from build123d import *

# Parameters (mm, degrees)
SKETCH_1_W                = 58.8
SKETCH_1_H                = 32
EXTRUDE_1_DEPTH           = 41.5
HOLE_WIZARD_1_D           = 3.2
HOLE_WIZARD_1_CBORE_D     = 6
HOLE_WIZARD_1_CBORE_DEPTH = 32.5
SKETCH_8_R                = 2.6
CUT_EXTRUDE_6_DEPTH       = 33.5
SKETCH_10_W               = 58.8
SKETCH_10_H               = 41.5
EXTRUDE_2_DEPTH           = 3
SKETCH_18_R               = 2.6
CUT_EXTRUDE_14_DEPTH      = 4
SKETCH_19_W               = 20
SKETCH_19_H               = 20
SKETCH_19_R               = 3
CUT_EXTRUDE_15_DEPTH      = 22
SKETCH_20_R               = 3
CUT_EXTRUDE_16_DEPTH      = 5
CUT_EXTRUDE_17_DEPTH      = 6
SKETCH_22_W               = 27.4
SKETCH_22_H               = 21.5
CUT_EXTRUDE_18_DEPTH      = 36
SKETCH_23_R               = 2.6
CUT_EXTRUDE_19_DEPTH      = 16
CUT_EXTRUDE_20_DEPTH      = 6
SKETCH_25_W               = 20
SKETCH_25_H               = 17
SKETCH_25_R               = 2.6
CUT_EXTRUDE_21_DEPTH      = 0.1
SKETCH_27_W               = 17
SKETCH_27_H               = 20.1
CUT_EXTRUDE_22_DEPTH      = 0.1
SKETCH_28_R               = 2.6
CUT_EXTRUDE_23_DEPTH      = 39.7
SKETCH_29_R               = 4.5
SKETCH_29_R_2             = 2.6
CUT_EXTRUDE_24_DEPTH      = 5
SKETCH_30_R               = 2.6
CUT_EXTRUDE_25_DEPTH      = 36.0000001
SKETCH_31_R               = 2.6
EXTRUDE_3_DEPTH           = 35
SKETCH_32_W               = 20.1
SKETCH_32_H               = 17
SKETCH_32_R               = 2.6
CUT_EXTRUDE_26_DEPTH      = 7
SKETCH_33_W               = 20.1
SKETCH_33_H               = 7
SKETCH_33_R               = 3
EXTRUDE_4_DEPTH           = 17
SKETCH_34_R               = 4.5
EXTRUDE_5_DEPTH           = 5
SKETCH_35_R               = 2.6
EXTRUDE_6_DEPTH           = 6.3
SKETCH_39_R               = 2.6
CUT_EXTRUDE_29_DEPTH      = 8
SKETCH_40_W               = 20.1
SKETCH_40_H               = 17
SKETCH_40_R               = 2.6
EXTRUDE_7_DEPTH           = 7.9
SKETCH_41_W               = 20.1
SKETCH_41_H               = 17
CUT_EXTRUDE_30_DEPTH      = 7.9
SKETCH_42_R               = 2.6
CUT_EXTRUDE_31_DEPTH      = 39.7
SKETCH_43_R               = 4.5
SKETCH_43_R_2             = 2.6
CUT_EXTRUDE_32_DEPTH      = 5.2
SKETCH_44_R               = 2.6
EXTRUDE_8_DEPTH           = 3
SKETCH_46_R               = 4.75
SKETCH_46_R_2             = 2.6
CUT_EXTRUDE_33_DEPTH      = 3


with BuildPart() as part:
    # 草图1 → 凸台-拉伸1 (new body)
    with BuildSketch(Plane.XY):
        with Locations((-0.739622642, 3.045283019)):
            Rectangle(SKETCH_1_W, SKETCH_1_H)
    extrude(amount=EXTRUDE_1_DEPTH)

    # 孔1 (through all)
    with Locations(Plane(origin=(11.760377358, 15.545283019, 0), x_dir=(-1, 0, 0), z_dir=(0, 0, -1))):
        with Locations((0, 0), (25, 0), (25, -25), (0, -25)):
            CounterBoreHole(HOLE_WIZARD_1_D / 2, HOLE_WIZARD_1_CBORE_D / 2, HOLE_WIZARD_1_CBORE_DEPTH)

    # 草图8 → 切除-拉伸6 (cut)
    with BuildSketch(Plane(origin=(0, 19.045283019, 0), x_dir=(1, 0, 0), z_dir=(0, 1, 0))):
        with Locations((-0.739622642, -31.5)):
            Circle(SKETCH_8_R)
    extrude(amount=-CUT_EXTRUDE_6_DEPTH, mode=Mode.SUBTRACT)

    # 草图10 → 凸台-拉伸2 (add)
    with BuildSketch(Plane.XZ.offset(12.954716981)):
        with Locations((-0.739622642, 20.75)):
            Rectangle(SKETCH_10_W, SKETCH_10_H)
    extrude(amount=EXTRUDE_2_DEPTH)

    # 草图18 → 切除-拉伸14 (cut, through all)
    with BuildSketch(Plane(origin=(0, -12.954716981, 0), x_dir=(1, 0, 0), z_dir=(0, 1, 0))):
        with Locations((-0.739622642, -31.5)):
            Circle(SKETCH_18_R)
    extrude(amount=-CUT_EXTRUDE_14_DEPTH, mode=Mode.SUBTRACT)

    # 草图19 → 切除-拉伸15 (cut)
    with BuildSketch(Plane(origin=(0, 0, 0), x_dir=(-1, 0, 0), z_dir=(0, 0, -1))):
        with Locations((20.139622642, 9.045283019)):
            Rectangle(SKETCH_19_W, SKETCH_19_H)
        with Locations((13.239622642, 15.545283019)):
            Circle(SKETCH_19_R, mode=Mode.SUBTRACT)
    extrude(amount=-CUT_EXTRUDE_15_DEPTH, mode=Mode.SUBTRACT)

    # 草图20 → 切除-拉伸16 (cut)
    with BuildSketch(Plane(origin=(0, 0, 0), x_dir=(-1, 0, 0), z_dir=(0, 0, -1))):
        Polygon((30.139622642, -15.954716981), (30.139622642, -0.954716981), (10.139622642, -0.954716981), (10.139622642, 19.045283019), (-28.660377358, 19.045283019), (-28.660377358, -15.954716981), align=None)
        with Locations((13.239622642, -9.454716981)):
            Circle(SKETCH_20_R, mode=Mode.SUBTRACT)
        with Locations((-11.760377358, -9.454716981)):
            Circle(SKETCH_20_R, mode=Mode.SUBTRACT)
        with Locations((-11.760377358, 15.545283019)):
            Circle(SKETCH_20_R, mode=Mode.SUBTRACT)
    extrude(amount=-CUT_EXTRUDE_16_DEPTH, mode=Mode.SUBTRACT)

    # 草图21 → 切除-拉伸17 (cut)
    with BuildSketch(Plane.XZ.offset(15.954716981)):
        Polygon((-30.139622642, 19.214629022), (-17.064744213, 5), (-30.139622642, 5), align=None)
    extrude(amount=-CUT_EXTRUDE_17_DEPTH, mode=Mode.SUBTRACT)

    # 草图22 → 切除-拉伸18 (cut, through all)
    with BuildSketch(Plane(origin=(0, 19.045283019, 0), x_dir=(1, 0, 0), z_dir=(0, 1, 0))):
        with Locations((14.960377358, -15.75)):
            Rectangle(SKETCH_22_W, SKETCH_22_H)
    extrude(amount=-CUT_EXTRUDE_18_DEPTH, mode=Mode.SUBTRACT)

    # 草图23 → 切除-拉伸19 (cut, through all)
    with BuildSketch(Plane(origin=(0, -0.954716981, 0), x_dir=(1, 0, 0), z_dir=(0, 1, 0))):
        with Locations((-20.139622642, -13.5)):
            Circle(SKETCH_23_R)
    extrude(amount=-CUT_EXTRUDE_19_DEPTH, mode=Mode.SUBTRACT)

    # 草图24 → 切除-拉伸20 (cut)
    with BuildSketch(Plane(origin=(0, -15.954716981, 0), x_dir=(-1, 0, 0), z_dir=(0, -1, 0))):
        with BuildLine():
            ThreePointArc((20.787086214, -9.046822379), (16.827633547, -16.546428767), (24.631280369, -13.22611889))
            Line((24.631280369, -13.22611889), (20.787086214, -9.046822379))
        make_face()
        with BuildLine():
            ThreePointArc((20.139622642, -16.1), (18.30114501, -11.661522369), (22.739622642, -13.5))
            ThreePointArc((22.739622642, -13.5), (21.978100273, -15.338477631), (20.139622642, -16.1))
        make_face(mode=Mode.SUBTRACT)
    extrude(amount=-CUT_EXTRUDE_20_DEPTH, mode=Mode.SUBTRACT)

    # 草图25 → 切除-拉伸21 (cut)
    with BuildSketch(Plane(origin=(0, -0.954716981, 0), x_dir=(1, 0, 0), z_dir=(0, 1, 0))):
        with Locations((-20.139622642, -13.5)):
            Rectangle(SKETCH_25_W, SKETCH_25_H)
        with Locations((-20.139622642, -13.5)):
            Circle(SKETCH_25_R, mode=Mode.SUBTRACT)
    extrude(amount=-CUT_EXTRUDE_21_DEPTH, mode=Mode.SUBTRACT)

    # 草图27 → 切除-拉伸22 (cut)
    with BuildSketch(Plane.ZY.offset(10.139622642)):
        with Locations((13.5, 8.995283019)):
            Rectangle(SKETCH_27_W, SKETCH_27_H)
    extrude(amount=-CUT_EXTRUDE_22_DEPTH, mode=Mode.SUBTRACT)

    # 草图28 → 切除-拉伸23 (cut, through all)
    with BuildSketch(Plane.ZY.offset(10.039622642)):
        with Locations((13.5, 8.995283019)):
            Circle(SKETCH_28_R)
    extrude(amount=-CUT_EXTRUDE_23_DEPTH, mode=Mode.SUBTRACT)

    # 草图29 → 切除-拉伸24 (cut)
    with BuildSketch(Plane(origin=(1.260377358, 0, 0), x_dir=(0, 0, -1), z_dir=(1, 0, 0))):
        with Locations((-13.5, 8.995283019)):
            Circle(SKETCH_29_R)
        with Locations((-13.5, 8.995283019)):
            Circle(SKETCH_29_R_2, mode=Mode.SUBTRACT)
    extrude(amount=-CUT_EXTRUDE_24_DEPTH, mode=Mode.SUBTRACT)

    # 草图30 → 切除-拉伸25 (cut, through all)
    with BuildSketch(Plane(origin=(0, 19.045283019, 0), x_dir=(1, 0, 0), z_dir=(0, 1, 0))):
        with Locations((-20.139622642, -31.5)):
            Circle(SKETCH_30_R)
    extrude(amount=-CUT_EXTRUDE_25_DEPTH, mode=Mode.SUBTRACT)

    # 草图31 → 凸台-拉伸3 (add, through all)
    with BuildSketch(Plane(origin=(0, 19.045283019, 0), x_dir=(1, 0, 0), z_dir=(0, 1, 0))):
        with Locations((-0.739622642, -31.5)):
            Circle(SKETCH_31_R)
    extrude(amount=-EXTRUDE_3_DEPTH)

    # 草图32 → 切除-拉伸26 (cut)
    with BuildSketch(Plane(origin=(0, -1.054716981, 0), x_dir=(1, 0, 0), z_dir=(0, 1, 0))):
        with Locations((-20.089622642, -13.5)):
            Rectangle(SKETCH_32_W, SKETCH_32_H)
        with Locations((-20.139622642, -13.5)):
            Circle(SKETCH_32_R, mode=Mode.SUBTRACT)
    extrude(amount=-CUT_EXTRUDE_26_DEPTH, mode=Mode.SUBTRACT)

    # 草图33 → 凸台-拉伸4 (add)
    with BuildSketch(Plane(origin=(0, 0, 22), x_dir=(-1, 0, 0), z_dir=(0, 0, -1))):
        with Locations((20.089622642, 15.545283019)):
            Rectangle(SKETCH_33_W, SKETCH_33_H)
        with Locations((13.239622642, 15.545283019)):
            Circle(SKETCH_33_R, mode=Mode.SUBTRACT)
    extrude(amount=EXTRUDE_4_DEPTH)

    # 草图34 → 凸台-拉伸5 (add)
    with BuildSketch(Plane(origin=(-3.739622642, 0, 0), x_dir=(0, 0, -1), z_dir=(1, 0, 0))):
        with Locations((-13.5, 8.995283019)):
            Circle(SKETCH_34_R)
    extrude(amount=EXTRUDE_5_DEPTH)

    # 草图35 → 凸台-拉伸6 (add)
    with BuildSketch(Plane.ZY.offset(3.739622642)):
        with Locations((13.5, 8.995283019)):
            Circle(SKETCH_35_R)
    extrude(amount=EXTRUDE_6_DEPTH)

    # 草图39 → 切除-拉伸29 (cut, through all)
    with BuildSketch(Plane.XZ.offset(-12.045283019)):
        with Locations((-20.139622642, 13.5)):
            Circle(SKETCH_39_R)
    extrude(amount=-CUT_EXTRUDE_29_DEPTH, mode=Mode.SUBTRACT)

    # 草图40 → 凸台-拉伸7 (add)
    with BuildSketch(Plane.XZ.offset(-12.045283019)):
        with Locations((-20.089622642, 13.5)):
            Rectangle(SKETCH_40_W, SKETCH_40_H)
        with Locations((-20.139622642, 13.5)):
            Circle(SKETCH_40_R, mode=Mode.SUBTRACT)
    extrude(amount=EXTRUDE_7_DEPTH)

    # 草图41 → 切除-拉伸30 (cut)
    with BuildSketch(Plane(origin=(0, -8.054716981, 0), x_dir=(1, 0, 0), z_dir=(0, 1, 0))):
        with Locations((-20.089622642, -13.5)):
            Rectangle(SKETCH_41_W, SKETCH_41_H)
    extrude(amount=-CUT_EXTRUDE_30_DEPTH, mode=Mode.SUBTRACT)

    # 草图42 → 切除-拉伸31 (cut, through all)
    with BuildSketch(Plane.ZY.offset(10.039622642)):
        with Locations((13.5, -5.854716981)):
            Circle(SKETCH_42_R)
    extrude(amount=-CUT_EXTRUDE_31_DEPTH, mode=Mode.SUBTRACT)

    # 草图43 → 切除-拉伸32 (cut)
    with BuildSketch(Plane(origin=(1.260377358, 0, 0), x_dir=(0, 0, -1), z_dir=(1, 0, 0))):
        with Locations((-13.5, -5.854716981)):
            Circle(SKETCH_43_R)
        with Locations((-13.5, -5.854716981)):
            Circle(SKETCH_43_R_2, mode=Mode.SUBTRACT)
    extrude(amount=-CUT_EXTRUDE_32_DEPTH, mode=Mode.SUBTRACT)

    # 草图44 → 凸台-拉伸8 (add)
    with BuildSketch(Plane(origin=(0, 19.045283019, 0), x_dir=(1, 0, 0), z_dir=(0, 1, 0))):
        Polygon((1.260377358, -5), (-30.139622642, -5), (-30.139622642, -41.5), (28.660377358, -41.5), (28.660377358, -26.5), (1.260377358, -26.5), align=None)
        with Locations((-20.139622642, -13.5)):
            Circle(SKETCH_44_R, mode=Mode.SUBTRACT)
        with Locations((-20.139622642, -31.5)):
            Circle(SKETCH_44_R, mode=Mode.SUBTRACT)
    extrude(amount=EXTRUDE_8_DEPTH)

    # 草图46 → 切除-拉伸33 (cut)
    with BuildSketch(Plane(origin=(0, 22.045283019, 0), x_dir=(1, 0, 0), z_dir=(0, 1, 0))):
        with Locations((-20.139622642, -31.5)):
            Circle(SKETCH_46_R)
        with Locations((-20.139622642, -31.5)):
            Circle(SKETCH_46_R_2, mode=Mode.SUBTRACT)
    extrude(amount=-CUT_EXTRUDE_33_DEPTH, mode=Mode.SUBTRACT)


solid = part.part
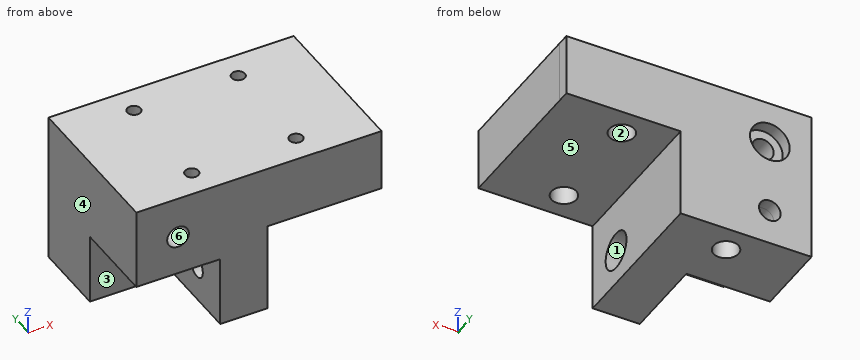
Work out the finished part from the listing and answer in its coordinate system (mm). Face numbers are marked on the shaded views. A direction names the side the tool comes from. Coordinates: 2 decimals unless noted, no trailing zeros. Write each loop counter-clockwise with the first axis right and the second up, starting at its lowest first coordinate (ties: lowest second). Pieces come first, ordered by that corner, then holes. Notation, with made-up numbers: M 63,25.5 L 121,25.5 A35 ccw 121,60.5 Z; hole C 57.5,67 d3. An arc over 180 degrees is marked long. Answer as CSV lines item,"result". Start each with the question number.
Item 1: Consider L1, parallel to X at y = 20, z = 13.5; L2, parallel to Y at x = -11.5, z = 28; L3, parallel to Z at x = -11, y = 16.5. Determine where each line is inside the solid, lowest interval first.
Item 2: Determine the mould class of the marked faces 4, 5 and 6 for opening direction X: released by +X, released by -X, zero draft, split by the parting line, or undercut.
Item 3: A tool of negligible diameter and unlimited length cuts with its end or side. For the marked faces 1, 2 and 3, from which of +Z, -Z, +X, -X, +Y, -Y can it reach the whole face along a straight path? Write none if from no direction.
Item 4: Section C-C on y = 2.5 is taken. Write down the section's boundary in (x, z).
Item 5: Section D-D on z = 31.5 is taken. Write down the section's boundary in (x, y), and give its area (3 significant figures).
Item 6: Flat-ended cylindrical pins translate along their axes: P1, Ø1.5, axis at x = 8.5, y = 1.5, coming from the -Z side; P2, Ø1.9, axis at x = -13.24, y = 15.55, coming from the -Z side; P3, Ø18.5, axis at y = -6, z = 10.5, coming from the -X side; P4, Ø1.8, axis at x = 12.5, y = 14.5, coming from the -Z side. Find the tip coordinate at first contact, or state that the pin passes through.
Item 7: Section B-B on z = 13.5 is taken. Write down the section's boundary in (x, y), and give its area (3 significant figures).
Item 8: Section A-A on y = -4 is taken. Write down the section's boundary in (x, z), and give its area (3 significant figures).
Checks:
1,L1,"x = -30.14 to -22.74, -17.54 to 1.26"
1,L2,"y = -15.95 to -11.9, -7.01 to 13.1, 17.99 to 22.05"
1,L3,"z = 32.5 to 41.5"
2,face 4,"released by -X"
2,face 5,"zero draft"
2,face 6,"undercut"
3,face 1,"+X"
3,face 2,"-Z"
3,face 3,"-Z, -X, -Y"
4,outline,"M -30.14,22 L -10.04,22 L -10.04,5 L 1.26,5 L 1.26,26.5 L 28.66,26.5 L 28.66,41.5 L -30.14,41.5 Z; hole C -20.14,31.5 d5.2"
5,outline,"M -30.14,-15.95 L -22.74,-15.95 L -22.74,19.05 L -24.89,19.05 L -24.89,22.05 L -30.14,22.05 Z; M -17.54,-15.95 L 28.66,-15.95 L 28.66,22.05 L -15.39,22.05 L -15.39,19.05 L -17.54,19.05 Z; hole C -13.24,-9.45 d6; hole C -13.24,15.55 d6; hole C 11.76,-9.45 d6; hole C 11.76,15.55 d6"
5,area,"1,910 mm²"
6,P1,"stops at z = 26.5"
6,P2,"passes through"
6,P3,"stops at x = -10.04"
6,P4,"stops at z = 32.5"
7,outline,"M -30.14,4.15 L -22.74,4.15 L -22.74,22.05 L -30.14,22.05 Z; M -17.54,4.15 L -10.04,4.15 L -10.04,-3.25 L -3.94,-3.25 L -3.94,-1.35 L 1.26,-1.35 L 1.26,22.05 L -17.54,22.05 Z; M -10.04,-15.95 L 1.26,-15.95 L 1.26,-10.35 L -3.94,-10.35 L -3.94,-8.45 L -10.04,-8.45 Z; hole C -13.24,15.55 d6"
7,area,"589 mm²"
8,outline,"M -30.14,22 L -10.04,22 L -10.04,15.32 L -3.94,15.32 L -3.94,17.6 L 1.26,17.6 L 1.26,26.5 L 28.66,26.5 L 28.66,41.5 L -30.14,41.5 Z; M -10.04,5 L 1.26,5 L 1.26,9.4 L -3.94,9.4 L -3.94,11.68 L -10.04,11.68 Z; hole C -20.14,31.5 d5.2"
8,area,"1,130 mm²"
